Verification items for the finished model (mm, model axes). A direction names the side the tool comes from. Round coordinates to 2 decimals unless told otherwise and drop trailing zeros. Write each loop counter-clockwise with the first axis right and the second up, starting at its lowest first coordinate (ties: lowest second). Pieces come first, ordered by that corner, then holes. Notation, with made-up numbers: M 4,1.25 L 42,1.25 A20 ccw 42,23.25 Z; hole C 48,-3.75 d4. An arc over 180 degrees is marked long. One line per question, with ' | ' between items.
from build123d import *

# Parameters (mm, degrees)
TOP_DEPTH                 = 2.54
SKETCH13_W                = 12.446
SKETCH13_H                = 1.27
BODY_TABS_DEPTH           = 1.27
BODY_TABS_DRAFT           = 7
BODY_TABS_PROFILE_2_DEPTH = 1.27
BODY_TABS_PROFILE_2_DRAFT = 7
SKETCH14_W                = 6.985
SKETCH14_H                = 1.905
FLAT_HEAD_HOLE_DEPTH      = 73.383371188
SKETCH15_W                = 6.35
SKETCH15_H                = 0.762
HOLD_GRPOVES_DEPTH        = 0.381
HOLD_FILLETS_R            = 0.381


with BuildPart() as part:
    # Sketch2 → top (new body)
    with BuildSketch(Plane(origin=(0, 0, 0), x_dir=(1, 0, 0), z_dir=(0, 1, 0))):
        with BuildLine():
            Line((-25.3365, -60.2615), (25.3365, -60.2615))
            ThreePointArc((25.3365, -60.2615), (34.316756121, -56.541756121), (38.0365, -47.5615))
            Line((38.0365, -47.5615), (38.0365, 47.5615))
            ThreePointArc((38.0365, 47.5615), (34.316756121, 56.541756121), (25.3365, 60.2615))
            Line((25.3365, 60.2615), (-25.3365, 60.2615))
            ThreePointArc((-25.3365, 60.2615), (-34.316756121, 56.541756121), (-38.0365, 47.5615))
            Line((-38.0365, 47.5615), (-38.0365, -47.5615))
            ThreePointArc((-38.0365, -47.5615), (-34.316756121, -56.541756121), (-25.3365, -60.2615))
        make_face()
    extrude(amount=TOP_DEPTH)


with BuildPart() as body_tabs_tool:
    # Sketch13 → Body Tabs (with draft: the straight prism first)
    with BuildSketch(Plane(origin=(0, 0, -60.2615), x_dir=(-1, 0, 0), z_dir=(0, 0, -1))):
        with Locations((-12.7, 0.635)):
            Rectangle(SKETCH13_W, SKETCH13_H)
    extrude(amount=BODY_TABS_DEPTH)
    # Body Tabs: the draft: its side faces are tilted about the plane it starts from
    body_tabs_sides = [body_tabs_tool.faces().sort_by_distance(p)[0] for p in [
        (12.7, 0, -60.8965),
        (6.477, 0.635, -60.8965),
        (12.7, 1.27, -60.8965),
        (18.923, 0.635, -60.8965),
    ]]
    draft(body_tabs_sides, Plane(origin=(0, 0, -60.2615), x_dir=(-1, 0, 0), z_dir=(0, 0, -1)), BODY_TABS_DRAFT)


with BuildPart() as part_1:
    add(part.part)

    # Body Tabs: add body_tabs_tool
    add(body_tabs_tool.part)


with BuildPart() as body_tabs_profile_2_tool:
    # Sketch13 → Body Tabs profile 2 (with draft: the straight prism first)
    with BuildSketch(Plane(origin=(0, 0, -60.2615), x_dir=(-1, 0, 0), z_dir=(0, 0, -1))):
        with Locations((12.7, 0.635)):
            Rectangle(SKETCH13_W, SKETCH13_H)
    extrude(amount=BODY_TABS_PROFILE_2_DEPTH)
    # Body Tabs profile 2: the draft: its side faces are tilted about the plane it starts from
    body_tabs_profile_2_sides = [body_tabs_profile_2_tool.faces().sort_by_distance(p)[0] for p in [
        (-18.923, 0.635, -60.8965),
        (-12.7, 1.27, -60.8965),
        (-6.477, 0.635, -60.8965),
        (-12.7, 0, -60.8965),
    ]]
    draft(body_tabs_profile_2_sides, Plane(origin=(0, 0, -60.2615), x_dir=(-1, 0, 0), z_dir=(0, 0, -1)), BODY_TABS_PROFILE_2_DRAFT)


with BuildPart() as part_2:
    add(part_1.part)

    # Body Tabs profile 2: add body_tabs_profile_2_tool
    add(body_tabs_profile_2_tool.part)

    # Sketch14 → Flat Head Hole (cut, through all)
    with BuildSketch(Plane(origin=(0, 2.54, 0), x_dir=(1, 0, 0), z_dir=(0, 1, 0))):
        with Locations((0, -59.309)):
            Rectangle(SKETCH14_W, SKETCH14_H)
    extrude(amount=-FLAT_HEAD_HOLE_DEPTH, mode=Mode.SUBTRACT)

    # Sketch15 → Hold Grpoves (cut)
    with BuildSketch(Plane.XY.offset(60.2615)):
        with Locations((-9.525, 1.27)):
            Rectangle(SKETCH15_W, SKETCH15_H)
        with Locations((9.525, 1.27)):
            Rectangle(SKETCH15_W, SKETCH15_H)
    extrude(amount=-HOLD_GRPOVES_DEPTH, mode=Mode.SUBTRACT)

    # Hold Fillets
    hold_fillets_edges = [part_2.edges().sort_by_distance(p)[0] for p in [
        (9.525, 1.651, 59.8805),
        (9.525, 0.889, 59.8805),
        (-9.525, 0.889, 59.8805),
        (-9.525, 1.651, 59.8805),
    ]]
    fillet(hold_fillets_edges, radius=HOLD_FILLETS_R - 0.0001)  # a hair under: the kernel refuses the full size


solid = part_2.part
1. Thickness scan on line 1 (Z direction, x = 19, y = 1.35); line 2 (Z direction, x = -31.5, y = 0.95); line 3 (X direction, y = 2.2, z = -51.5). Record the ranges inside material, lowest first.
Results:
line 1: z = -60.26 to 60.26 | line 2: z = -58.67 to 58.67 | line 3: x = -37.41 to 37.41
2. Section check A-A, the plane x = -33. Record the cut outline in (y, z).
Results:
outline: M 0,-57.69 L 2.54,-57.69 L 2.54,57.69 L 0,57.69 Z
3. Section check B-B, the plane x = 33.5. Record the cut outline in (y, z), then the cut area to 3 significant figures.
Results:
outline: M 0,-57.29 L 2.54,-57.29 L 2.54,57.29 L 0,57.29 Z | area: 291 mm2
4. Tool access check on faces 1 (the face through (-1, 2.54, -1)), 2 (the face through (0, 2, -60.262)). Record the directions out of +Z, -Z, +X, -X, +Y, -Y that give a thin tool (end or side, any length) a straight path to the whole face; none if there is none.
Results:
face 1: +Z, -Z, +X, -X, +Y | face 2: -Z, +Y
5. Go/stop test with flat-tipped pins: P1, Ø0.8, axis at x = -1, y = 1.5, coming from the -Z side; P2, Ø1.5, axis at y = 1, z = 59.5, coming from the +X side. Record where each tip stops, or that it passes through.
Results:
P1: stops at z = -60.26 | P2: stops at x = 31.35
6. Mould release check, pull along X, two halves, no side actions. Record for faces 3 (the face through (0, 1, 58.356)), 4 (the face through (-38.036, 1, -1)), 5 (the face through (-15, 1, 60.262)): pulls with the +X half, pulls with the -X half, needs draft (parallel to the pull), parting line crosses it, or undercut.
Results:
face 3: undercut | face 4: pulls with the -X half | face 5: needs draft
